Read the model definition and answer for the solid it produces. Units are mm, in the model's axes. Coordinates: 2 decimals unless noted, no trailing zeros. Write each loop counter-clockwise with the first axis right and the second up, starting at its lowest first coordinate (ties: lowest second). Pieces come first, ordered by that corner, then holes. Notation, with made-up numbers: (4.5, 15) - (45.5, 15) arc R20 cw to (45.5, 26) - close; hole circle Ø1 at (-12.5, -16.75). An arc over 180 degrees is marked (long way). Return JSON: item names as keys, results as strings.
```python
from build123d import *

# Parameters (mm, degrees)
SKETCH1_W              = 25.4
SKETCH1_H              = 25.4
SKETCH1_W_2            = 19.05
SKETCH1_H_2            = 19.05
BOSS_EXTRUDE1_DEPTH    = 762
F_10_CLEARANCE_HOLE1_D = 5.1054
CUT_EXTRUDE1_REACH     = 764.846
SKETCH5_R              = 9.525


with BuildPart() as part:
    # Sketch1 → Boss-Extrude1 (new body)
    with BuildSketch(Plane.XY):
        with Locations((-12.7, 12.7)):
            Rectangle(SKETCH1_W, SKETCH1_H)
        with Locations((-12.7, 12.7)):
            Rectangle(SKETCH1_W_2, SKETCH1_H_2, mode=Mode.SUBTRACT)
    extrude(amount=BOSS_EXTRUDE1_DEPTH)

    # #10 Clearance Hole1 (through all)
    with Locations(Plane(origin=(0, 25.4, 0), x_dir=(1, 0, 0), z_dir=(0, 1, 0))):
        with Locations((-12.7, -749.3), (-12.7, -736.6), (-12.7, -723.9), (-12.7, -38.1), (-12.7, -25.4), (-12.7, -12.7)):
            Hole(F_10_CLEARANCE_HOLE1_D / 2)

    # Cut-Extrude1: up to this face of the body (flat: up to its plane)
    cut_extrude1_end = Plane(part.part.faces().sort_by_distance((0, 12.7, 381))[0])
    # Sketch5 → Cut-Extrude1 (cut, up to the picked face)
    with BuildSketch(Plane.ZY.offset(25.4), mode=Mode.PRIVATE) as cut_extrude1_sk1:
        with Locations(Location((50.8, 12.7, 0), (0, 0, 270))):
            Circle(SKETCH5_R)
    cut_extrude1_tool1 = split(extrude(cut_extrude1_sk1.sketch, amount=-CUT_EXTRUDE1_REACH, mode=Mode.PRIVATE), bisect_by=cut_extrude1_end, keep=Keep.BOTH, mode=Mode.PRIVATE)
    # Sketch5 → Cut-Extrude1 (cut, up to the picked face)
    with BuildSketch(Plane.ZY.offset(25.4), mode=Mode.PRIVATE) as cut_extrude1_sk2:
        with Locations(Location((711.2, 12.7, 0), (0, 0, 270))):
            Circle(SKETCH5_R)
    cut_extrude1_tool2 = split(extrude(cut_extrude1_sk2.sketch, amount=-CUT_EXTRUDE1_REACH, mode=Mode.PRIVATE), bisect_by=cut_extrude1_end, keep=Keep.BOTH, mode=Mode.PRIVATE)
    # Sketch5 → Cut-Extrude1 (cut, up to the picked face)
    with BuildSketch(Plane.ZY.offset(25.4), mode=Mode.PRIVATE) as cut_extrude1_sk3:
        with Locations(Location((504.825, 12.7, 0), (0, 0, 270))):
            Circle(SKETCH5_R)
    cut_extrude1_tool3 = split(extrude(cut_extrude1_sk3.sketch, amount=-CUT_EXTRUDE1_REACH, mode=Mode.PRIVATE), bisect_by=cut_extrude1_end, keep=Keep.BOTH, mode=Mode.PRIVATE)
    # Sketch5 → Cut-Extrude1 (cut, up to the picked face)
    with BuildSketch(Plane.ZY.offset(25.4), mode=Mode.PRIVATE) as cut_extrude1_sk4:
        with Locations(Location((257.175, 12.7, 0), (0, 0, 270))):
            Circle(SKETCH5_R)
    cut_extrude1_tool4 = split(extrude(cut_extrude1_sk4.sketch, amount=-CUT_EXTRUDE1_REACH, mode=Mode.PRIVATE), bisect_by=cut_extrude1_end, keep=Keep.BOTH, mode=Mode.PRIVATE)
    add(cut_extrude1_tool1.solids().sort_by(Axis((-25.4, 12.7, 50.8), (1, 0, 0)))[0], mode=Mode.SUBTRACT)
    add(cut_extrude1_tool2.solids().sort_by(Axis((-25.4, 12.7, 711.2), (1, 0, 0)))[0], mode=Mode.SUBTRACT)
    add(cut_extrude1_tool3.solids().sort_by(Axis((-25.4, 12.7, 504.825), (1, 0, 0)))[0], mode=Mode.SUBTRACT)
    add(cut_extrude1_tool4.solids().sort_by(Axis((-25.4, 12.7, 257.175), (1, 0, 0)))[0], mode=Mode.SUBTRACT)


solid = part.part
```
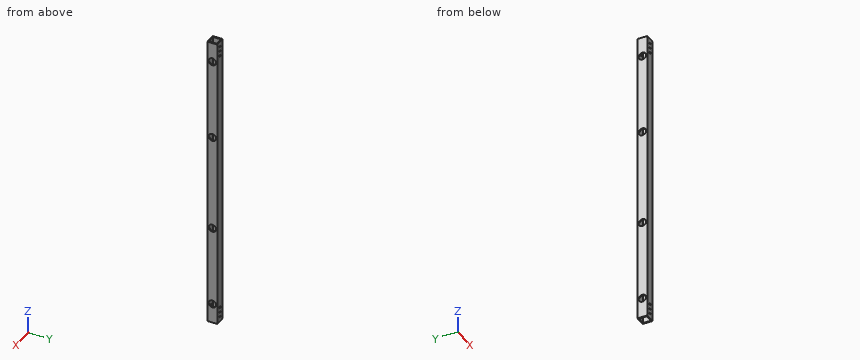
(1) Flat-ended cylindrical pins translate along their axes: P1, Ø15, axis at y = 15, z = 725, coming from the +X side; P2, Ø3, axis at x = -12.7, z = 723.9, coming from the -Y side. Find the tip coordinate at first contact, or state that the pin passes through.
Answer:
{"P1": "x = 0", "P2": "through"}
(2) A cutting plane is placed at A-A (z = 445.5). Determine the outline of the cut face in (x, y) (3 decimals), and give its area (3 significant figures).
Answer:
{"outline": "(-25.4, 0) - (0, 0) - (0, 25.4) - (-25.4, 25.4) - close; hole (-22.225, 3.175) - (-3.175, 3.175) - (-3.175, 22.225) - (-22.225, 22.225) - close", "area": "282 mm²"}
(3) A cutting plane is placed at B-B (y = 7.25). State how many separate pieces and enclosed holes the cut face has, and give its area (3 significant figures).
Answer:
{"separate pieces": "10", "enclosed holes": "0", "area": "4,440 mm²"}
(4) Straight lines are drawn through the part: line 1 (Z direction, x = -1.45, y = 12.7) (3 decimals); line 2 (X direction, y = 18, z = 124) (3 decimals); line 3 (Y direction, x = -8, z = 392) (3 decimals). For each, find the intervals that lie inside material, in ascending order. Write a range as from..to.
Answer:
{"line 1": "0..41.275, 60.325..247.65, 266.7..495.3, 514.35..701.675, 720.725..762", "line 2": "-25.4..-22.225, -3.175..0", "line 3": "0..3.175, 22.225..25.4"}
